Part model, mm, in its own coordinate system. Give positions to 0.01 mm unless a question says otherwise; leave off trailing zeros. Order: outer loops, then holes, each group sorted by start corner. A loop starts at its lowest first (then second) coordinate and runs counter-clockwise, first axis right, second up.
Autodesk Inventor part; units mm, degrees
ref_plane "YZ Plane" through (0, 0, 0) normal (1, 0, 0) x (0, 1, 0)
ref_plane "XZ Plane" through (0, 0, 0) normal (0, 1, 0) x (-1, 0, 0)
ref_plane "XY Plane" through (0, 0, 0) normal (0, 0, 1) x (1, 0, 0)
sketch "Sketch1" plane through (0, 0, 0) normal (0, 1, 0) x (-1, 0, 0)
  line L0 (0, 0) -> (169, 0)
  line L1 (169, 0) -> (169, -30)
  line L2 (169, -30) -> (0, -30)
  line L3 (0, -30) -> (0, 0)
  dimension "d0" = 169
  dimension "d1" = 30
extrude "Extrusion1" add sketch "Sketch1" along normal blind 4
sketch "Sketch2" plane through (0, 0, 0) normal (0, -1, 0) x (1, 0, 0)
  line L0 (0, 0) -> (0, -30)
  line L1 (0, -15) -> (-169, -15) construction
  line L2 (-169, -30) -> (-169, 0)
  line L3 (-84.5, -15) -> (-84.5, 52.7002) construction
  point P0 (-161.5, -15)
  point P1 (-7.5, -15)
  dimension "d6" = 154
hole "Hole1" at (-161.5, 0, -15) at (-7.5, 0, -15) direction (0, 1, 0) diameter 4 end through all
sketch "Sketch3" plane through (0, 0, 0) normal (0, -1, 0) x (1, 0, 0)
  line L0 (-169, -30) -> (-169, 0) construction
  line L1 (-169, -15) -> (0, -15) construction
  line L2 (0, 0) -> (0, -30) construction
  line L3 (-169, -4.25) -> (0, -4.25)
  line L4 (-169, -4.25) -> (-169, -15)
  line L5 (0, -4.25) -> (0, -15)
  line L6 (-169, -25.75) -> (0, -25.75)
  line L7 (-169, -25.75) -> (-169, -15)
  line L8 (0, -25.75) -> (0, -15)
  dimension "d15" = 21.5
extrude "Extrusion2" [suppressed]
properties part number "ballastBar" material "Steel"
Item 1: Drill centre lines: probe 1 along X at (y, z) = (3, -15); probe 2 along Z at (x, y) = (-7.5, 2.3); probe 3 along X at (y, z) = (3.6, -14.25). Where is each one in solid material? Low to high.
Item 2: Band-saw the part on A-A on x = -7.5. List the corners of the cut face in (y, z), plus the area to 3 significant figures.
Item 3: Pull direction X, two halves, no side cores. Call faces 1 (the face through (-169, 2, -15)), 2 (the face through (-159.726, 2.028, -15.923)), 3 (the face through (-83, 2, 0)): released by +X, released by -X, zero draft, split by the parting line, or undercut.
Working result:
1. probe 1: x = -169 to -163.5, -159.5 to -9.5, -5.5 to 0
1. probe 2: z = -30 to -17, -13 to 0
1. probe 3: x = -169 to -163.35, -159.65 to -9.35, -5.65 to 0
2. outline: (0, -30) - (4, -30) - (4, -17) - (0, -17) - close; (0, -13) - (4, -13) - (4, 0) - (0, 0) - close
2. area: 104 mm2
3. face 1: released by -X
3. face 2: undercut
3. face 3: zero draft
